Autodesk Inventor part; units mm, degrees
ref_plane "YZ Plane" through (0, 0, 0) normal (1, 0, 0) x (0, 1, 0)
ref_plane "XZ Plane" through (0, 0, 0) normal (0, 1, 0) x (-1, 0, 0)
ref_plane "XY Plane" through (0, 0, 0) normal (0, 0, 1) x (1, 0, 0)
sketch "Sketch1" plane through (0, 0, 0) normal (0, 0, 1) x (1, 0, 0)
  circle A0 centre (0, 0) radius 30
  circle A1 centre (0, 100) radius 30
  line L0 (-20, 0) -> (20, 0)
  line L1 (20, 0) -> (20, 100)
  line L2 (20, 100) -> (-20, 100)
  line L3 (-20, 100) -> (-20, 0)
  point P0 (20, 77.6393)
  point P1 (-20, 77.6393)
  point P2 (-20, 22.3607)
  point P3 (20, 22.3607)
  dimension "d0" = 60
  dimension "d1" = 60
  dimension "d2" = 40
extrude "Extrusion1" add sketch "Sketch1" along normal blind 20
sketch "Sketch2" plane through (0, 0, 20) normal (0, 0, 1) x (1, 0, 0)
  circle A0 centre (0, 0) radius 10
  dimension "d5" = 20
extrude "Extrusion2" cut sketch "Sketch2" against normal blind 16
sketch "Sketch3" plane through (0, 0, 4) normal (0, 0, 1) x (1, 0, 0)
  circle A0 centre (0, 0) radius 1
  circle A1 centre (5, 0) radius 1
  circle A2 centre (-5, 0) radius 1
  dimension "d11" = 2
  dimension "d12" = 2
  dimension "d13" = 2
extrude "Extrusion3" cut sketch "Sketch3" against normal blind 28.45
sketch "Sketch4" plane through (0, 0, 0) normal (0, 0, -1) x (-1, 0, 0)
  line L0 (0, 100) -> (10, 100)
  line L1 (10, 100) -> (10, 70)
  line L2 (10, 70) -> (0, 70)
  line L3 (0, 70) -> (0, 100)
  line L4 (0, 100) -> (-10, 100)
  line L5 (-10, 100) -> (-10, 70)
  line L6 (-10, 70) -> (0, 70)
  line L7 (0, 70) -> (0, 100)
  line L8 (10, 100) -> (-10, 100)
  line L9 (-10, 100) -> (-10, 110.5)
  line L10 (-10, 110.5) -> (10, 110.5)
  line L11 (10, 110.5) -> (10, 100)
  point P0 (0, 0)
  dimension "d16" = 10
  dimension "d17" = 30
  dimension "d18" = 10
  dimension "d19" = 10.5
extrude "Extrusion4" cut sketch "Sketch4" against normal blind 16
sketch "Sketch5" plane through (0, 0, 0) normal (0, 0, -1) x (-1, 0, 0)
  line L0 (10, 110.5) -> (10, 70)
  line L1 (10, 110.5) -> (-10, 110.5)
  line L2 (-10, 110.5) -> (-10, 118.1)
  line L3 (-10, 118.1) -> (10, 118.1)
  line L4 (10, 118.1) -> (10, 110.5)
  line L5 (10, 70) -> (-10, 70)
  line L6 (-10, 70) -> (-10, 62.4)
  line L7 (-10, 62.4) -> (10, 62.4)
  line L8 (10, 62.4) -> (10, 70)
  line L9 (-10, 110.5) -> (10, 110.5)
  line L10 (10, 110.5) -> (-10, 110.5)
  line L11 (-10, 110.5) -> (-10, 114.6)
  line L12 (-10, 114.6) -> (10, 114.6)
  line L13 (10, 114.6) -> (10, 110.5)
  line L14 (10, 70) -> (-10, 70)
  line L15 (-10, 70) -> (-10, 65.9)
  line L16 (-10, 65.9) -> (10, 65.9)
  line L17 (10, 65.9) -> (10, 70)
  line L18 (0, 110.5) -> (5, 110.5)
  line L19 (5, 110.5) -> (5, 114.6)
  line L20 (5, 114.6) -> (0, 114.6)
  line L21 (0, 114.6) -> (0, 110.5)
  line L22 (0, 110.5) -> (-5, 110.5)
  line L23 (-5, 110.5) -> (-5, 114.6)
  line L24 (-5, 114.6) -> (0, 114.6)
  line L25 (0, 114.6) -> (0, 110.5)
  line L26 (0, 70) -> (5, 70)
  line L27 (5, 70) -> (5, 65.9)
  line L28 (5, 65.9) -> (0, 65.9)
  line L29 (0, 65.9) -> (0, 70)
  line L30 (0, 70) -> (-5, 70)
  line L31 (-5, 70) -> (-5, 65.9)
  line L32 (-5, 65.9) -> (0, 65.9)
  line L33 (0, 65.9) -> (0, 70)
  point P0 (0, 0)
  dimension "d22" = 7.6
  dimension "d23" = 7.6
  dimension "d24" = 4.1
  dimension "d25" = 4.1
  dimension "d26" = 5
  dimension "d27" = 5
  dimension "d28" = 5
  dimension "d29" = 5
extrude "Extrusion5" cut sketch "Sketch5" against normal blind 10
sketch "Sketch6" plane through (0, 0, 10) normal (0, 0, -1) x (-1, 0, 0)
  line L0 (10, 110.5) -> (10, 70)
  line L1 (-10, 62.4) -> (-10, 118.1)
  line L2 (10, 110.5) -> (-10, 110.5)
  line L3 (-10, 110.5) -> (-10, 114.6)
  line L4 (-10, 114.6) -> (10, 114.6)
  line L5 (10, 114.6) -> (10, 110.5)
  line L6 (10, 70) -> (-10, 70)
  line L7 (-10, 62.4) -> (-10, 70)
  line L8 (10, 70) -> (-10, 70)
  line L9 (-10, 70) -> (-10, 65.9)
  line L10 (-10, 65.9) -> (10, 65.9)
  line L11 (10, 65.9) -> (10, 70)
  line L12 (-10, 110.5) -> (10, 110.5)
  line L13 (0, 114.6) -> (5, 114.6)
  line L14 (5, 114.6) -> (5, 110.5)
  line L15 (5, 110.5) -> (0, 110.5)
  line L16 (0, 110.5) -> (0, 114.6)
  line L17 (0, 110.5) -> (-5, 110.5)
  line L18 (-5, 110.5) -> (-5, 114.6)
  line L19 (-5, 114.6) -> (0, 114.6)
  line L20 (0, 114.6) -> (0, 110.5)
  line L21 (0, 70) -> (5, 70)
  line L22 (5, 70) -> (5, 65.9)
  line L23 (5, 65.9) -> (0, 65.9)
  line L24 (0, 65.9) -> (0, 70)
  line L25 (0, 70) -> (-5, 70)
  line L26 (-5, 70) -> (-5, 65.9)
  line L27 (-5, 65.9) -> (0, 65.9)
  line L28 (0, 65.9) -> (0, 70)
  circle A0 centre (5, 114.6) radius 1.35
  circle A1 centre (-5, 114.6) radius 1.35
  circle A2 centre (5, 65.9) radius 1.35
  circle A3 centre (-5, 65.9) radius 1.35
  point P0 (0, 0)
  dimension "d32" = 4.1
  dimension "d33" = 4.1
  dimension "d34" = 5
  dimension "d35" = 5
  dimension "d36" = 2.7
  dimension "d37" = 2.7
  dimension "d38" = 2.7
  dimension "d39" = 2.7
extrude "Extrusion6" cut sketch "Sketch6" against normal blind 8 contours A0 L4 L14 | L14 L4 A0 | L4 A0 | A2 L10 L22 | L22 L10 A2 | A2 L10 | A1 L4 L18 | L18 L4 A1 | L4 A1 | A3 L10 L26 | L26 L10 A3 | A3 L10
sketch "Sketch7" plane through (0, 0, 20) normal (0, 0, 1) x (1, 0, 0)
  circle A0 centre (0, 100) radius 10
  point P0 (0, 0)
  dimension "d50" = 20
extrude "Extrusion7" cut sketch "Sketch7" against normal blind 4
sketch "Sketch8" plane through (0, 0, 0) normal (0, 0, -1) x (-1, 0, 0)
  line L0 (20, 77.6393) -> (20, 22.3607)
  arc A0 (20, 77.6393) -> (-20, 77.6393) centre (0, 100) ccw
  line L1 (20, 22.3607) -> (-20, 22.3607)
  line L2 (-20, 22.3607) -> (-20, 77.6393)
  line L3 (-20, 77.6393) -> (20, 77.6393)
  line L4 (20, 77.6393) -> (20, 22.3607)
  line L5 (10, 118.1) -> (10, 62.4)
  line L6 (10, 77.6393) -> (-10, 77.6393)
  line L7 (-10, 77.6393) -> (-10, 47.6393)
  line L8 (-10, 47.6393) -> (10, 47.6393)
  line L9 (10, 47.6393) -> (10, 77.6393)
  line L10 (-10, 22.3607) -> (10, 22.3607)
  line L11 (10, 22.3607) -> (10, 52.3607)
  line L12 (10, 52.3607) -> (-10, 52.3607)
  line L13 (-10, 52.3607) -> (-10, 22.3607)
  line L14 (20, 77.6393) -> (10, 52.3607)
  line L15 (10, 47.6393) -> (20, 22.3607)
  line L16 (-20, 77.6393) -> (-10, 52.3607)
  line L17 (-10, 47.6393) -> (-20, 22.3607)
  point P0 (0, 0)
  dimension "d53" = 20
  dimension "d54" = 30
  dimension "d55" = 30
extrude "Extrusion8" cut sketch "Sketch8" against normal blind 72.2 contours L0 L15 L9 L14 | L16 L7 L17 L2
sketch "Sketch9" plane through (0, 0, 20) normal (0, 0, 1) x (1, 0, 0)
  circle A0 centre (0, 0) radius 1
  circle A1 centre (0, 0) radius 10
extrude "Extrusion9" add sketch "Sketch9" against normal blind 20
sketch "Sketch10" plane through (0, 0, 0) normal (0, 0, -1) x (-1, 0, 0)
  circle A0 centre (0, 0) radius 1
  circle A1 centre (0, 0) radius 10
  dimension "d60" = 20
extrude "Extrusion10" cut sketch "Sketch10" against normal blind 16
sketch "Sketch11" plane through (0, 0, 16) normal (0, 0, -1) x (-1, 0, 0)
  circle A0 centre (0, 5) radius 1
  circle A1 centre (0, -5) radius 1
  point P0 (0, 0)
  dimension "d63" = 2
  dimension "d64" = 2
extrude "Extrusion11" cut sketch "Sketch11" against normal blind 22.1
chamfer "Chamfer2" distance 12 angle 45 1 edges at (10, 0, 0)
thread "Thread5"
thread "Thread6"
thread "Thread7"
thread "Thread8"
sketch "Sketch12" plane through (0, 0, 16) normal (0, 0, -1) x (-1, 0, 0)
  circle A0 centre (0, 0) radius 1
  circle A1 centre (0, 0) radius 1.5
  dimension "d78" = 3
extrude "Extrusion12" cut sketch "Sketch12" against normal blind 10
properties part number "2ndArm"
Input: part model. Units: mm. Frame: model coordinates. A direction names the side the tool comes from. Give positions to 0.01 mm unless a question says otherwise; leave off trailing zeros. Order: outer loops, then holes, each group sorted by start corner. A loop starts at its lowest first (then second) coordinate and runs counter-clockwise, first axis right, second up.
1. Reachability of faces 4 (the cylindrical face through (1.5, 0.07, 17.97)), 5 (the flat face through (10, 50, 10)), 6 (the flat face through (-15, 65, 10)), 7 (the flat face through (0, 62.4, 5)) from +Z, -Z, +X, -X, +Y, -Y: full face, straight path, thin tool, end or side. Return the list, or none.
Derived:
face 4: +Z, -Z
face 5: +Z, -Z, +X
face 6: +Z, -Z, -X
face 7: -Z
2. Material intervals for L1, parallel to Y at x = 0, z = 19.2; L2, parallel to X at y = 100, z = 18.55; L3, parallel to X at y = 65.9, z = 15, sorted ascending.
Derived:
L1: y = -30 to -6, -4 to -1.5, 1.5 to 4, 6 to 90, 110 to 130
L2: x = -30 to -10, 10 to 30
L3: x = -15.36 to -6.35, -3.65 to 3.65, 6.35 to 15.36
3. Section A-A on y = 94.5. Return the cut outline in (x, z).
Derived:
outline: (-29.49, 0) - (-10, 0) - (-10, 16) - (-8.35, 16) - (-8.35, 20) - (-29.49, 20) - close; (8.35, 16) - (10, 16) - (10, 0) - (29.49, 0) - (29.49, 20) - (8.35, 20) - close
4. Section B-B on y = 50.5. Return the cut outline in (x, z).
Derived:
outline: (-10, 0) - (10, 0) - (10, 20) - (-10, 20) - close
5. Pin query (flat end, axial travel): pin 1 (4 mm diameter, centred on x = 17, z = 11.5, fed in from -Y); pin 2 (2.5 mm diameter, centred on y = 49.5, z = 9, fed in from +X); pin 3 (6 mm diameter, centred on y = -9, z = 5, fed in from +X). Return the tip coordinate at first contact, or that it passes through.
Derived:
pin 1: stops at y = -25.98
pin 2: stops at x = 10
pin 3: stops at x = 29.39
6. Mould query, pull axis X, two halves, no side actions, for faces 1 (the flat face through (-15, 35, 10)), 2 (the flat face through (0, 118.1, 5)), 3 (the flat face through (15, 35, 10)). Classes: released by +X, released by -X, zero draft, split by the parting line, or undercut.
Derived:
face 1: released by -X
face 2: undercut
face 3: released by +X
